Check sheet for the modelled part. Datum: model origin and axes. Units: mm. A direction names the side the tool comes from. Round coordinates to 2 decimals unless told otherwise and drop trailing zeros. Loops run counter-clockwise (first coordinate to the right, second up) from the corner with the lowest first, then second, coordinate; pieces in that order, holes last. Notation, with made-up numbers: (-3, -15.75) -> (22, -15.75) arc R22 cw to (22, -6.75) -> close; hole circle Ø7 at (28, 34.5). An arc over 180 degrees is marked (long way). Use one line per item in the form item = value. Start each with the question number.
(1) Sectioned sample at B-B (z = 74). Record the cut outline in (x, y).
(2) Material ranges on probe 1 along Z at (x, y) = (0.5, 13.75); probe 2 along X at (y, z) = (11.5, 46); probe 3 along X at (y, z) = (11.65, 55), recorded low to high. Write a range as [from, to].
(3) Go/stop test with flat-tipped pins: pin 1 (3 mm diameter, centred on x = -7, y = 14, fed in from -Z); pin 2 (3.5 mm diameter, centred on y = 12.5, z = 2, fed in from +X); pin 3 (2 mm diameter, centred on x = -26.16, z = 28.84, fed in from -Y); pin 4 (4 mm diameter, centred on x = -2, y = 12.5, fed in from -Z). Record where each tip stops, or that it passes through.
(4) Sectioned sample at C-C (z = 55). Record the cut outline in (x, y).
(5) Draft check along X on faces 1 (the flat face through (18, 16.7, 14)), 2 (the cylindrical face through (26.238, 10.672, 30.535)), 3 (the flat face through (-12, 10, 2)). Enter one of: released by +X, released by -X, zero draft, split by the parting line, or undercut.
(6) Set-up check for faces 4 (the flat face through (20, 13, 8)), 5 (the flat face through (-26, 12.7, 32)), 6 (the flat face through (-4, 13, 2)), 7 (the flat face through (8, 11.7, 2)): record each of +Z, -Z, +X, -X, +Y, -Y from which the full face is reachable in a straight line by a thin tool's end or side.
(7) Sectioned sample at D-D (z = 14.5). Record the cut outline in (x, y).
(8) Sectioned sample at A-A (x = 0). Record the cut outline in (y, z).
from build123d import *

# Parameters (mm, degrees)
SKETCH_1_R                   = 26.5
EXTRUDE_1_DEPTH              = 5
HOLE_WIZARD_M4_1_AT_2_COUNT  = 2
HOLE_WIZARD_M4_1_AT_2_PITCH  = 39.424388736
HOLE_WIZARD_M4_1_AT_3_COUNT  = 2
HOLE_WIZARD_M4_1_AT_3_PITCH  = 39.424388736
HOLE_WIZARD_M4_1_AT_4_COUNT  = 2
HOLE_WIZARD_M4_1_AT_4_PITCH  = 18.383894388
HOLE_WIZARD_M4_1_AT_5_COUNT  = 2
HOLE_WIZARD_M4_1_AT_5_PITCH  = 43.5
HOLE_WIZARD_M4_1_AT_6_COUNT  = 2
HOLE_WIZARD_M4_1_AT_6_PITCH  = 39.424388736
HOLE_WIZARD_M4_1_AT_7_COUNT  = 2
HOLE_WIZARD_M4_1_AT_7_PITCH  = 18.383894388
EXTRUDE_1604_DEPTH           = 8
SKETCH_8_R                   = 34.5
CUT_EXTRUDE_1696_DEPTH       = 119.962346984
HOLE_WIZARD_M3_1_D           = 3.4
HOLE_WIZARD_M3_1_CBORE_D     = 6.5
HOLE_WIZARD_M3_1_CBORE_DEPTH = 3
SKETCH_11_R                  = 26.5
CUT_EXTRUDE_1_DEPTH          = 5
SKETCH_12_R                  = 44
CUT_EXTRUDE_6_DEPTH          = 4


with BuildPart() as part:
    # 草图1 → 凸台-拉伸1 (new body)
    with BuildSketch(Plane.XY):
        Circle(SKETCH_1_R)
    extrude(amount=EXTRUDE_1_DEPTH)

    # 草图3 → M4 六角凹头盖的柱孔1 (revolve, cut)
    with BuildSketch(Plane(origin=(21.75, 0, 5), x_dir=(0, -1, 0), z_dir=(1, 0, 0))):
        Polygon((0, 0), (0, 5), (2.25, 5), (2.25, 4), (4, 4), (4, 0), align=None)
    hole_wizard_m4_1 = revolve(axis=Axis((21.75, 0, 11.35), (0, 0, -1)), mode=Mode.SUBTRACT)

    # M4 六角凹头盖的柱孔1 at 2: M4 六角凹头盖的柱孔1 ×2
    with Locations(*[Vector(-0.9063077870366496, 0.4226182617407002, 0) * (i * HOLE_WIZARD_M4_1_AT_2_PITCH) for i in range(1, HOLE_WIZARD_M4_1_AT_2_COUNT)]):
        add(hole_wizard_m4_1, mode=Mode.SUBTRACT)

    # M4 六角凹头盖的柱孔1 at 3: M4 六角凹头盖的柱孔1 ×2
    with Locations(*[Vector(-0.9063077870125524, 0.42261826179237694, 0) * (i * HOLE_WIZARD_M4_1_AT_3_PITCH) for i in range(1, HOLE_WIZARD_M4_1_AT_3_COUNT)]):
        add(hole_wizard_m4_1, mode=Mode.SUBTRACT)

    # M4 六角凹头盖的柱孔1 at 4: M4 六角凹头盖的柱孔1 ×2
    with Locations(*[Vector(-0.42261826172613215, 0.9063077870434428, 0) * (i * HOLE_WIZARD_M4_1_AT_4_PITCH) for i in range(1, HOLE_WIZARD_M4_1_AT_4_COUNT)]):
        add(hole_wizard_m4_1, mode=Mode.SUBTRACT)

    # M4 六角凹头盖的柱孔1 at 5: M4 六角凹头盖的柱孔1 ×2
    with Locations(*[(-i * HOLE_WIZARD_M4_1_AT_5_PITCH, 0, 0) for i in range(1, HOLE_WIZARD_M4_1_AT_5_COUNT)]):
        add(hole_wizard_m4_1, mode=Mode.SUBTRACT)

    # M4 六角凹头盖的柱孔1 at 6: M4 六角凹头盖的柱孔1 ×2
    with Locations(*[Vector(-0.9063077870125524, -0.42261826179237694, 0) * (i * HOLE_WIZARD_M4_1_AT_6_PITCH) for i in range(1, HOLE_WIZARD_M4_1_AT_6_COUNT)]):
        add(hole_wizard_m4_1, mode=Mode.SUBTRACT)

    # M4 六角凹头盖的柱孔1 at 7: M4 六角凹头盖的柱孔1 ×2
    with Locations(*[Vector(-0.42261826172613215, -0.9063077870434428, 0) * (i * HOLE_WIZARD_M4_1_AT_7_PITCH) for i in range(1, HOLE_WIZARD_M4_1_AT_7_COUNT)]):
        add(hole_wizard_m4_1, mode=Mode.SUBTRACT)

    # 草图5 → Extrude 1604 (add)
    with BuildSketch(Plane.XZ.offset(-8.7)):
        with BuildLine():
            Line((-20, 5), (-20, 11.365151541))
            ThreePointArc((-20, 11.365151541), (0, 103), (20, 11.365151541))
            Line((20, 11.365151541), (20, 5))
            Line((20, 5), (-20, 5))
        make_face()
    extrude(amount=-EXTRUDE_1604_DEPTH)

    # 草图8 → Cut-Extrude 1696 (cut, through all)
    with BuildSketch(Plane.XZ.offset(-8.7)):
        with Locations(Location((0, 55, 0), (0, 0, 270))):
            Circle(SKETCH_8_R)
    extrude(amount=-CUT_EXTRUDE_1696_DEPTH, mode=Mode.SUBTRACT)

    # M3 六角凹头盖的柱孔1 (through all)
    with Locations(Plane(origin=(-9.576304669, 16.7, 19.260744427), x_dir=(0, 0, 1), z_dir=(0, 1, 0))):
        with Locations((0, 0), (0, 19.152609338), (9.576304669, 35.739255573), (26.162950904, 45.315560242), (45.315560242, 45.315560242), (62.358629164, 36.19567826), (71.478511143, 19.152609339), (71.478511146, 0), (61.902206477, -16.586646235), (9.576304669, -16.586646235), (26.162950904, -26.162950904), (45.315560242, -26.162950904)):
            CounterBoreHole(HOLE_WIZARD_M3_1_D / 2, HOLE_WIZARD_M3_1_CBORE_D / 2, HOLE_WIZARD_M3_1_CBORE_DEPTH)

    # 草图11 → 切除-拉伸1 (cut)
    with BuildSketch(Plane.XY):
        Circle(SKETCH_11_R)
        Polygon((-4, 14.7), (4, 14.7), (4, 11.7), (12, 11.7), (12, 8.7), (-12, 8.7), (-12, 11.7), (-4, 11.7), align=None, mode=Mode.SUBTRACT)
    extrude(amount=CUT_EXTRUDE_1_DEPTH, mode=Mode.SUBTRACT)

    # 草图12 → 切除-拉伸6 (cut)
    with BuildSketch(Plane(origin=(0, 16.7, 0), x_dir=(1, 0, 0), z_dir=(0, 1, 0))):
        with Locations(Location((0, -55, 0), (0, 0, 270))):
            Circle(SKETCH_12_R)
    extrude(amount=-CUT_EXTRUDE_6_DEPTH, mode=Mode.SUBTRACT)


solid = part.part
Checks:
q1.outline = (-44.08, 8.7) -> (-28.8, 8.7) -> (-28.8, 12.7) -> (-39.69, 12.7) -> (-39.69, 16.7) -> (-44.08, 16.7) -> close; (28.8, 8.7) -> (44.08, 8.7) -> (44.08, 16.7) -> (39.69, 16.7) -> (39.69, 12.7) -> (28.8, 12.7) -> close
q2.probe_1 = [0, 11], [99, 103]
q2.probe_2 = [-47.15, -37.34], [-34.14, -33.31], [33.31, 34.14], [37.34, 47.15]
q2.probe_3 = [-48, -34.5], [34.5, 48]
q3.pin_1 = 5
q3.pin_2 = 12
q3.pin_3 = through
q3.pin_4 = 0
q4.outline = (-48, 8.7) -> (-34.5, 8.7) -> (-34.5, 12.7) -> (-44, 12.7) -> (-44, 16.7) -> (-48, 16.7) -> close; (34.5, 8.7) -> (48, 8.7) -> (48, 16.7) -> (44, 16.7) -> (44, 12.7) -> (34.5, 12.7) -> close
q5.face_1 = zero draft
q5.face_2 = undercut
q5.face_3 = released by -X
q6.face_4 = -Z, +X, +Y, -Y
q6.face_5 = +Y
q6.face_6 = -Z, -X, +Y
q6.face_7 = -Z, +X, +Y
q7.outline = (-25.76, 8.7) -> (25.76, 8.7) -> (25.76, 16.7) -> (17.2, 16.7) -> (17.2, 12.7) -> (-17.2, 12.7) -> (-17.2, 16.7) -> (-25.76, 16.7) -> close
q8.outline = (8.7, 0) -> (14.7, 0) -> (14.7, 5) -> (16.7, 5) -> (16.7, 11) -> (12.7, 11) -> (12.7, 20.5) -> (8.7, 20.5) -> close; (8.7, 89.5) -> (12.7, 89.5) -> (12.7, 99) -> (16.7, 99) -> (16.7, 103) -> (8.7, 103) -> close
